```python
from build123d import *

# Parameters (mm, degrees)
SKETCH1_W                   = 15.24
SKETCH1_H                   = 8.1
BOSS_EXTRUDE1_DEPTH         = 10
CUT_EXTRUDE1_DEPTH          = 20.946618761
CUT_EXTRUDE2_DEPTH          = 20.946618761
SKETCH4_W                   = 1
SKETCH4_H                   = 0.66
BOSS_EXTRUDE2_DEPTH         = 3.5
CUT_EXTRUDE3_REACH          = 20.747
LPATTERN1_COUNT             = 3
LPATTERN1_PITCH             = 5.08
SKETCH6_W                   = 2.6
SKETCH6_H                   = 1.9
CUT_EXTRUDE4_DEPTH          = 1.7
CHAMFER1_SIZE               = 0.6
CHAMFER1_SIZE2              = 1.648486452
CHAMFER2_SIZE               = 0.6
CHAMFER2_SIZE2              = 1.648486452
CHAMFER3_SIZE               = 1.6
CHAMFER4_SIZE               = 0.9
CHAMFER4_SIZE2              = 1.62364298
LPATTERN2_COUNT             = 3
LPATTERN2_PITCH             = 5.08
CHAMFER1_OF_LPATTERN2_SIZE2 = 1.648486452
CHAMFER1_OF_LPATTERN2_SIZE  = 0.6
CHAMFER2_OF_LPATTERN2_SIZE2 = 1.648486452
CHAMFER2_OF_LPATTERN2_SIZE  = 0.6
CHAMFER3_OF_LPATTERN2_SIZE  = 1.6
CHAMFER4_OF_LPATTERN2_SIZE2 = 1.62364298
CHAMFER4_OF_LPATTERN2_SIZE  = 0.9
SKETCH7_R                   = 1.8
CUT_EXTRUDE5_DEPTH          = 1
SKETCH8_W                   = 0.6
SKETCH8_H                   = 3.54964787
CUT_EXTRUDE6_DEPTH          = 1
LPATTERN3_COUNT             = 3
LPATTERN3_PITCH             = 5.08


with BuildPart() as part:
    # Sketch1 → Boss-Extrude1 (new body)
    with BuildSketch(Plane(origin=(0, 0, 0), x_dir=(1, 0, 0), z_dir=(0, 1, 0))):
        with Locations((7.62, 4.05)):
            Rectangle(SKETCH1_W, SKETCH1_H)
    extrude(amount=BOSS_EXTRUDE1_DEPTH)

    # Sketch2 → Cut-Extrude1 (cut, through all)
    with BuildSketch(Plane(origin=(15.24, 0, 0), x_dir=(0, 0, -1), z_dir=(1, 0, 0))):
        Polygon((0, 10), (1.5, 10), (0.8, 5.7), (0, 5.7), align=None)
    extrude(amount=-CUT_EXTRUDE1_DEPTH, mode=Mode.SUBTRACT)

    # Sketch3 → Cut-Extrude2 (cut, through all)
    with BuildSketch(Plane(origin=(15.24, 0, 0), x_dir=(0, 0, -1), z_dir=(1, 0, 0))):
        Polygon((8.1, 3.8), (6.4, 10), (8.1, 10), align=None)
    extrude(amount=-CUT_EXTRUDE2_DEPTH, mode=Mode.SUBTRACT)

    # Sketch4 → Boss-Extrude2 (add)
    with BuildSketch(Plane.XZ):
        with Locations((2.54, -4.05)):
            Rectangle(SKETCH4_W, SKETCH4_H)
    boss_extrude2 = extrude(amount=BOSS_EXTRUDE2_DEPTH)

    # Sketch5 → Cut-Extrude3 (cut, up to next)
    with BuildSketch(Plane.XY.offset(-3.72), mode=Mode.PRIVATE) as cut_extrude3_sk1:
        Polygon((2.04, -2.643369181), (2.29, -3.5), (2.04, -3.5), align=None)
    cut_extrude3_tool1 = extrude(cut_extrude3_sk1.sketch, amount=-CUT_EXTRUDE3_REACH, mode=Mode.PRIVATE) & part.part
    # Sketch5 → Cut-Extrude3 (cut, up to next)
    with BuildSketch(Plane.XY.offset(-3.72), mode=Mode.PRIVATE) as cut_extrude3_sk2:
        Polygon((2.79, -3.5), (3.04, -3.5), (3.04, -2.643369181), align=None)
    cut_extrude3_tool2 = extrude(cut_extrude3_sk2.sketch, amount=-CUT_EXTRUDE3_REACH, mode=Mode.PRIVATE) & part.part
    cut_extrude3_1 = cut_extrude3_tool1.solids().sort_by_distance((2.123333, -3.214456, -3.72))[0]
    add(cut_extrude3_1, mode=Mode.SUBTRACT)
    cut_extrude3_2 = cut_extrude3_tool2.solids().sort_by_distance((2.956667, -3.214456, -3.72))[0]
    add(cut_extrude3_2, mode=Mode.SUBTRACT)
    cut_extrude3 = cut_extrude3_1 + cut_extrude3_2  # Cut-Extrude3 as one shape, for the pattern or mirror that repeats it

    # LPattern1: Boss-Extrude2, Cut-Extrude3 ×3
    with Locations(*[(i * LPATTERN1_PITCH, 0, 0) for i in range(1, LPATTERN1_COUNT)]):
        add(boss_extrude2)
        add(cut_extrude3, mode=Mode.SUBTRACT)

    # Sketch6 → Cut-Extrude4 (cut)
    with BuildSketch(Plane.XY):
        with Locations((2.54, 2.75)):
            Rectangle(SKETCH6_W, SKETCH6_H)
    cut_extrude4 = extrude(amount=-CUT_EXTRUDE4_DEPTH, mode=Mode.SUBTRACT)

    # Chamfer1
    chamfer1_edges = [part.edges().sort_by_distance(p)[0] for p in [
        (1.24, 2.75, 0),
    ]]
    chamfer1_side = [part.faces().sort_by_distance(p)[0] for p in [
        (7.926307978, 2.856029685, 0),
    ]]
    chamfer(chamfer1_edges, length=CHAMFER1_SIZE, length2=CHAMFER1_SIZE2, reference=chamfer1_side[0])

    # Chamfer2
    chamfer2_edges = [part.edges().sort_by_distance(p)[0] for p in [
        (3.84, 2.75, 0),
    ]]
    chamfer2_side = [part.faces().sort_by_distance(p)[0] for p in [
        (8.024891816, 2.85752587, 0),
    ]]
    chamfer(chamfer2_edges, length=CHAMFER2_SIZE, length2=CHAMFER2_SIZE2, reference=chamfer2_side[0])

    # Chamfer3
    chamfer3_edges = [part.edges().sort_by_distance(p)[0] for p in [
        (2.54, 3.7, 0),
    ]]
    chamfer(chamfer3_edges, length=CHAMFER3_SIZE)

    # Chamfer4
    chamfer4_edges = [part.edges().sort_by_distance(p)[0] for p in [
        (2.54, 1.8, 0),
    ]]
    chamfer4_side = [part.faces().sort_by_distance(p)[0] for p in [
        (8.53838843, 2.723450413, 0),
    ]]
    chamfer(chamfer4_edges, length=CHAMFER4_SIZE, length2=CHAMFER4_SIZE2, reference=chamfer4_side[0])

    # LPattern2: Cut-Extrude4 ×3
    with Locations(*[(i * LPATTERN2_PITCH, 0, 0) for i in range(1, LPATTERN2_COUNT)]):
        add(cut_extrude4, mode=Mode.SUBTRACT)

    # Chamfer1 of LPattern2
    chamfer1_of_lpattern2_edges = [part.edges().sort_by_distance(p)[0] for p in [
        (6.32, 2.75, 0),
        (11.4, 2.75, 0),
    ]]
    chamfer(chamfer1_of_lpattern2_edges, length=CHAMFER1_OF_LPATTERN2_SIZE, length2=CHAMFER1_OF_LPATTERN2_SIZE2)

    # Chamfer2 of LPattern2
    chamfer2_of_lpattern2_edges = [part.edges().sort_by_distance(p)[0] for p in [
        (8.92, 2.75, 0),
        (14, 2.75, 0),
    ]]
    chamfer(chamfer2_of_lpattern2_edges, length=CHAMFER2_OF_LPATTERN2_SIZE, length2=CHAMFER2_OF_LPATTERN2_SIZE2)

    # Chamfer3 of LPattern2
    chamfer3_of_lpattern2_edges = [part.edges().sort_by_distance(p)[0] for p in [
        (7.62, 3.7, 0),
        (12.7, 3.7, 0),
    ]]
    chamfer(chamfer3_of_lpattern2_edges, length=CHAMFER3_OF_LPATTERN2_SIZE)

    # Chamfer4 of LPattern2
    chamfer4_of_lpattern2_edges = [part.edges().sort_by_distance(p)[0] for p in [
        (7.62, 1.8, 0),
        (12.7, 1.8, 0),
    ]]
    chamfer(chamfer4_of_lpattern2_edges, length=CHAMFER4_OF_LPATTERN2_SIZE, length2=CHAMFER4_OF_LPATTERN2_SIZE2)

    # Sketch7 → Cut-Extrude5 (cut)
    with BuildSketch(Plane(origin=(0, 10, 0), x_dir=(1, 0, 0), z_dir=(0, 1, 0))):
        with Locations(Location((12.7, 3.95, 0), (0, 0, 270))):
            Circle(SKETCH7_R)
    cut_extrude5 = extrude(amount=-CUT_EXTRUDE5_DEPTH, mode=Mode.SUBTRACT)

    # Sketch8 → Cut-Extrude6 (cut)
    with BuildSketch(Plane(origin=(0, 9, 0), x_dir=(1, 0, 0), z_dir=(0, 1, 0))):
        with Locations((12.7, 3.95)):
            Rectangle(SKETCH8_W, SKETCH8_H)
    cut_extrude6 = extrude(amount=-CUT_EXTRUDE6_DEPTH, mode=Mode.SUBTRACT)

    # LPattern3: Cut-Extrude5, Cut-Extrude6 ×3
    with Locations(*[(-i * LPATTERN3_PITCH, 0, 0) for i in range(1, LPATTERN3_COUNT)]):
        add(cut_extrude5, mode=Mode.SUBTRACT)
        add(cut_extrude6, mode=Mode.SUBTRACT)


solid = part.part
```
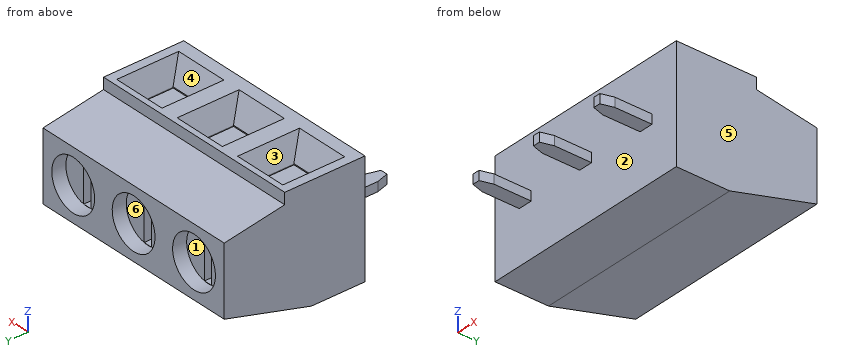
Could you check a few things on this model? Use its own coordinates, in mm. Face numbers are marked on the shaded views. A direction names the side the tool comes from. Coordinates: 2 decimals unless noted, no trailing zeros. Loops run counter-clockwise (first coordinate to the right, second up) from the corner with the lowest first, then second, coordinate; pieces in that order, holes last.
1) Imagine slicing it at C-C (y = 2). List the corners of the cut face in (x, z) for me.
Reported:
outline: (0, -8.1) - (15.24, -8.1) - (15.24, 0) - (14.6, 0) - (14, -1.65) - (14, -1.7) - (11.4, -1.7) - (11.4, -1.65) - (10.8, 0) - (9.52, 0) - (8.92, -1.65) - (8.92, -1.7) - (6.32, -1.7) - (6.32, -1.65) - (5.72, 0) - (4.44, 0) - (3.84, -1.65) - (3.84, -1.7) - (1.24, -1.7) - (1.24, -1.65) - (0.64, 0) - (0, 0) - close
2) Imagine slicing it at D-D (z = -5). List the corners of the cut face in (x, y) for me, and give its area (3 significant figures).
Reported:
outline: (0, 0) - (15.24, 0) - (15.24, 10) - (14.16, 10) - (14.16, 9) - (13, 9) - (13, 8) - (12.4, 8) - (12.4, 9) - (11.24, 9) - (11.24, 10) - (9.08, 10) - (9.08, 9) - (7.92, 9) - (7.92, 8) - (7.32, 8) - (7.32, 9) - (6.16, 9) - (6.16, 10) - (4, 10) - (4, 9) - (2.84, 9) - (2.84, 8) - (2.24, 8) - (2.24, 9) - (1.08, 9) - (1.08, 10) - (0, 10) - close
area: 142 mm2
3) Thinking about a two-plate mould opening in Z: for the marked faces 1, 2 and 3, which applies, released by +Z, released by -Z, zero draft, split by the parting line, or undercut?
Reported:
face 1: undercut
face 2: zero draft
face 3: released by +Z
4) Which directions (+Z, -Z, +X, -X, +Y, -Y) give clear straight access to the entire face, cutting with the end or side of a thin tool? Please do the marked faces 4, 5 and 6.
Reported:
face 4: +Z
face 5: +Z, -Z, +X, +Y, -Y
face 6: +Y
5) Imagine slicing it at A-A (y = -0.25). List the corners of the cut face in (x, z) for me, and give its area (3 significant figures).
Reported:
outline: (2.04, -4.38) - (3.04, -4.38) - (3.04, -3.72) - (2.04, -3.72) - close; (7.12, -4.38) - (8.12, -4.38) - (8.12, -3.72) - (7.12, -3.72) - close; (12.2, -4.38) - (13.2, -4.38) - (13.2, -3.72) - (12.2, -3.72) - close
area: 1.98 mm2
6) Please list where these lines run through material, in increasing order: line 1 along X through (y, z) = (9.45, -3.95); line 2 along X through (y, z) = (9.25, -5); line 3 along Y through (x, z) = (4, -1.75).
Reported:
line 1: x = 0 to 0.74, 4.34 to 5.82, 9.42 to 10.9, 14.5 to 15.24
line 2: x = 0 to 1.08, 4 to 6.16, 9.08 to 11.24, 14.16 to 15.24
line 3: y = 0 to 10
7) Will these pins go through, and if not, where does the flat tip stop? pin 1 Ø2 at (x, y) = (2.5, 7) entering from +Z; pin 2 Ø0.8 at (x, y) = (2.5, -2.5) entering from -Z; pin 3 Ø0.8 at (x, z) = (6.5, -3.5) entering from +Y; pin 4 Ø1.5 at (x, z) = (2, -2.5) entering from +Y.
Reported:
pin 1: stops at z = -0.85
pin 2: stops at z = -4.38
pin 3: stops at y = 9
pin 4: stops at y = 10
